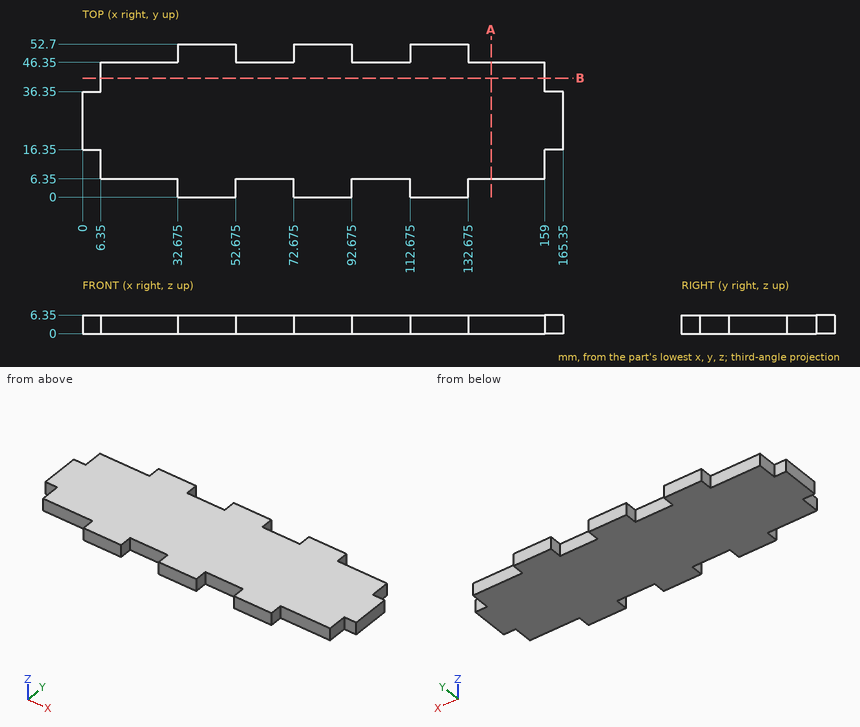
The figure shows three views and two pictorial views of one solid part (mm, origin at its lowest corner). Answer the questions. Round coordinates to 2 decimals unless told otherwise and drop trailing zeros. Write each loop counter-clockwise with the first axis right and the second up, starting at its lowest first coordinate (ties: lowest second). Pieces come first, ordered by that corner, then holes. Notation, with made-up numbers: M 58.5,43.25 L 96.5,43.25 A13 cw 96.5,61.25 Z; hole C 86.5,29.25 d8. An arc over 180 degrees is marked long. Use a Markdown table: item, result.
1) Straight lines are drawn through the part: line 1 along X through (y, z) = (48, 5) (3 decimals); line 2 along X through (y, z) = (14.5, 3); line 3 along Y through (x, z) = (94, 5.25). For each, find the intervals that lie inside material, in ascending order. Write a range as [from, to].
Answers follow:
| item | result |
|---|---|
| line 1 | x = [32.675, 52.675], [72.675, 92.675], [112.675, 132.675] |
| line 2 | x = [6.35, 159] |
| line 3 | y = [6.35, 46.35] |
2) The part is cut by section A-A (x = 140.5). Write down the section's boundary in (y, z), plus the area to 3 significant figures.
Answers follow:
| item | result |
|---|---|
| outline | M 6.35,0 L 46.35,0 L 46.35,6.35 L 6.35,6.35 Z |
| area | 254 mm2 |
3) The part is cut by section B-B (y = 41). Write down the section's boundary in (x, z), plus the area to 3 significant figures.
Answers follow:
| item | result |
|---|---|
| outline | M 6.35,0 L 159,0 L 159,6.35 L 6.35,6.35 Z |
| area | 969 mm2 |
4) Flat-ended cylindrical pins translate along their axes: pin 1 (1.9 mm diameter, centred on x = 16.5, z = 4.5, fed in from +Y); pin 2 (3 mm diameter, centred on y = 43.5, z = 2, fed in from -X); pin 3 (3 mm diameter, centred on x = 143.5, z = 1, fed in from -Y); pin 4 (10 mm diameter, centred on x = 104, y = 7, fed in from -Z). Find the tip coordinate at first contact, or state that the pin passes through.
Answers follow:
| item | result |
|---|---|
| pin 1 | stops at y = 46.35 |
| pin 2 | stops at x = 6.35 |
| pin 3 | stops at y = 6.35 |
| pin 4 | stops at z = 0 |
